```python
from build123d import *

# Parameters (mm, degrees)
F0_W     = 33.5
F0_H     = 20
F1_DEPTH = 30
F3_D     = 5
F4_D     = 7
F5_W     = 33.5
F5_H     = 14
F6_DEPTH = 30
F8_D     = 2


with BuildPart() as f1:
    # F0 (on Top) → F1 (new body)
    with BuildSketch(Plane.XY):
        Rectangle(F0_W, F0_H)
    extrude(amount=F1_DEPTH)

    # F3 (through all)
    with Locations(Plane.XY.offset(30)):
        with Locations((9.25, 0)):
            Hole(F3_D / 2)

    # F4 (through all)
    with Locations(Plane.XY.offset(30)):
        with Locations((-9.25, 0)):
            Hole(F4_D / 2)

    # F5 (on Top) → F6 (join)
    with BuildSketch(Plane.XY):
        with Locations((0, 17)):
            Rectangle(F5_W, F5_H)
    extrude(amount=F6_DEPTH)

    # F8 (through all)
    with Locations(Plane.YZ.offset(16.75)):
        with Locations((14, 15)):
            Hole(F8_D / 2)


solid = f1.part
```
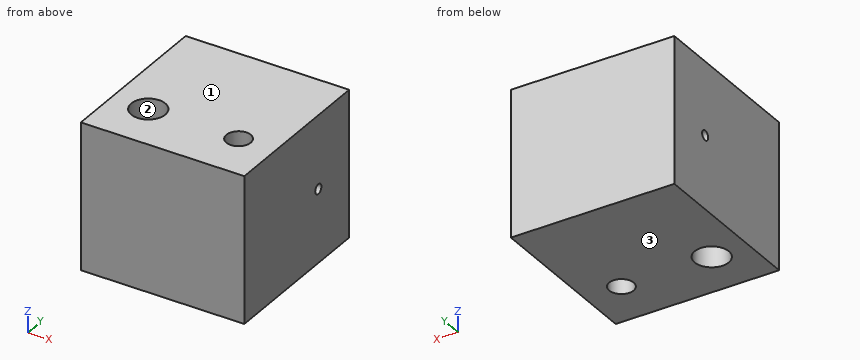
Geometry: final body of the model. Coordinates: model frame, mm. Face numbers are marked on the shaded views. Round coordinates to 2 decimals unless told otherwise and drop trailing zeros. Write each loop counter-clockwise with the first axis right and the second up, starting at its lowest first coordinate (ties: lowest second). Pieces come first, ordered by that corner, then holes. Notation, with made-up numbers: (80, 54) -> (135, 54) arc R27 cw to (135, 77) -> close; hole circle Ø1 at (-27.5, -16.5). An arc over 180 degrees is marked (long way). Use CSV: the item, a comma, the result in double quotes. Start each with the question number.
Q1. Section A-A (x = 9.25). Return loops of the section in (y, z), plus the area to 3 significant figures.
Q2. Line query: L1, parallel to Y at x = -9.25, z = 20.75; L2, parallel to Y at x = 9.25, z = 20; L3, parallel to Z at x = 5.5, y = 14. Output: solid intervals per line, ascending.
Q3. Section C-C (y = 14). Return loops of the section in (x, z).
Q4. Section D-D (z = 7.5). Return loops of the section in (x, y).
Q5. Section B-B (y = 0). Return loops of the section in (x, z).
Q6. Pull-direction query (Z, two-part tool) for the marked faces 1, 2 and 3; classes: pulls with the +Z half, pulls with the -Z half, needs draft (parallel to the pull), parting line crosses it, or undercut.
Result sheet:
1,outline,"(-10, 0) -> (-2.5, 0) -> (-2.5, 30) -> (-10, 30) -> close; (2.5, 0) -> (24, 0) -> (24, 30) -> (2.5, 30) -> close; hole circle Ø2 at (14, 15)"
1,area,"867 mm²"
2,L1,"-10 to -3.5, 3.5 to 24"
2,L2,"-10 to -2.5, 2.5 to 24"
2,L3,"0 to 14, 16 to 30"
3,outline,"(-16.75, 0) -> (16.75, 0) -> (16.75, 14) -> (-16.75, 14) -> close; (-16.75, 16) -> (16.75, 16) -> (16.75, 30) -> (-16.75, 30) -> close"
4,outline,"(-16.75, -10) -> (16.75, -10) -> (16.75, 24) -> (-16.75, 24) -> close; hole circle Ø7 at (-9.25, 0); hole circle Ø5 at (9.25, 0)"
5,outline,"(-16.75, 0) -> (-12.75, 0) -> (-12.75, 30) -> (-16.75, 30) -> close; (-5.75, 0) -> (6.75, 0) -> (6.75, 30) -> (-5.75, 30) -> close; (11.75, 0) -> (16.75, 0) -> (16.75, 30) -> (11.75, 30) -> close"
6,face 1,"pulls with the +Z half"
6,face 2,"needs draft"
6,face 3,"pulls with the -Z half"
